Build history of the part. All positions in model axes, mm. Face numbers are marked on the shaded views. Round coordinates to 2 decimals unless told otherwise and drop trailing zeros. Write each loop counter-clockwise with the first axis right and the second up, starting at its lowest first coordinate (ties: lowest second). Pieces come first, ordered by that corner, then holes.
Item 1: Band-saw the part on D-D, the plane x = -2.3. Write the cut outline in (y, z) (3 decimals), then the cut area to 3 significant figures.
Item 2: Band-saw the part on B-B, the plane z = 5. Write the cut outline in (x, y).
Item 3: Band-saw the part on C-C, the plane y = 3. Write the cut outline in (x, z) (3 decimals).
Item 4: Mould opens along Z. For the marked faces 1, 2 and 3 say: +Z half, -Z half, draft (parallel to the pull), parting line (faces both ways), or undercut.
Item 5: Band-saw the part on A-A, the plane x = 11. Write the cut outline in (y, z) (3 decimals).
Item 6: Drop a flat-ended pin along its axis: pin 1 Ø4.5 at (x, z) = (-2.3, 5) entering from -Y. Give the stop position or say it passes through.
Item 7: Wall check: probe 1 along Z at (x, y) = (-2.5, 3.5) (3 decimals); probe 2 along X at (y, z) = (3.25, 0); probe 3 along X at (y, z) = (2.75, 5). Give the ranges that are in metal, low to high.
```python
from build123d import *

# Parameters (mm, degrees)
SKETCH1_W             = 38
SKETCH1_H             = 19.05
BOSS_EXTRUDE1_DEPTH   = 6.35
M4X0_7_TAPPED_HOLE1_D = 3.3
M6X1_0_TAPPED_HOLE1_D = 5


with BuildPart() as part:
    # Sketch1 → Boss-Extrude1 (new body)
    with BuildSketch(Plane(origin=(0, 0, 0), x_dir=(1, 0, 0), z_dir=(0, 1, 0))):
        Rectangle(SKETCH1_W, SKETCH1_H)
    extrude(amount=BOSS_EXTRUDE1_DEPTH)

    # M4x0.7 Tapped Hole1 (through all)
    with Locations(Plane(origin=(-2.3, 6.35, -5), x_dir=(0, 0, 1), z_dir=(0, 1, 0))):
        with Locations((0, 0), (10, 0)):
            Hole(M4X0_7_TAPPED_HOLE1_D / 2)

    # M6x1.0 Tapped Hole1 (through all)
    with Locations(Plane(origin=(11, 6.35, 0), x_dir=(0, 0, 1), z_dir=(0, 1, 0))):
        with Locations((0, 0)):
            Hole(M6X1_0_TAPPED_HOLE1_D / 2)


solid = part.part
```
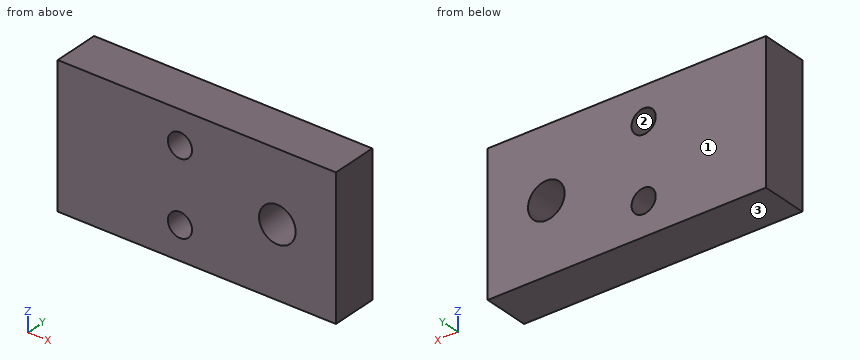
Results:
1. outline: (0, -9.525) - (6.35, -9.525) - (6.35, -6.65) - (0, -6.65) - close; (0, -3.35) - (6.35, -3.35) - (6.35, 3.35) - (0, 3.35) - close; (0, 6.65) - (6.35, 6.65) - (6.35, 9.525) - (0, 9.525) - close
1. area: 79.1 mm2
2. outline: (-19, 0) - (-3.95, 0) - (-3.95, 6.35) - (-19, 6.35) - close; (-0.65, 0) - (19, 0) - (19, 6.35) - (-0.65, 6.35) - close
3. outline: (-19, -9.525) - (19, -9.525) - (19, 9.525) - (-19, 9.525) - close; hole circle Ø3.3 at (-2.3, -5); hole circle Ø3.3 at (-2.3, 5); hole circle Ø5 at (11, 0)
4. face 1: draft
4. face 2: undercut
4. face 3: -Z half
5. outline: (0, -9.525) - (6.35, -9.525) - (6.35, -2.5) - (0, -2.5) - close; (0, 2.5) - (6.35, 2.5) - (6.35, 9.525) - (0, 9.525) - close
6. pin 1: stops at y = 0
7. probe 1: z = -9.525 to -6.638, -3.362 to 3.362, 6.638 to 9.525
7. probe 2: x = -19 to 8.5, 13.5 to 19
7. probe 3: x = -19 to -3.95, -0.65 to 19
